Could you check a few things on this model? Use its own coordinates, in mm. Face numbers are marked on the shaded views. A direction names the side the tool comes from. Give positions to 0.01 mm unless a question says otherwise; leave off trailing zeros. Loops run counter-clockwise (first coordinate to the right, second up) from the corner with the lowest first, then second, coordinate; pieces in that order, holes last. Notation, with made-up numbers: (-26.5, 70) - (10.5, 70) arc R27 cw to (10.5, 97) - close; hole circle Ø11 at (32.25, -12.5). An arc over 180 degrees is marked (long way). Write each question's results on one line, items separated by ' | '. Start each with the question number.
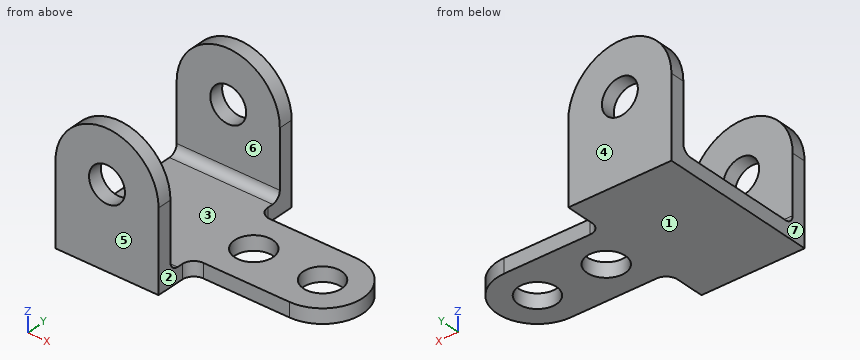
```python
from build123d import *

# Parameters (mm, degrees)
F0_R     = 9.94537
F1_DEPTH = 88.9
F3_DEPTH = 57.151
F4_R     = 10.5537
F5_DEPTH = 7.9375


with BuildPart() as f1:
    # F0 (on Front) → F1 (new body)
    with BuildSketch(Plane.XZ):
        with BuildLine():
            Line((28.575, 0), (28.575, 44.45))
            ThreePointArc((28.575, 44.45), (0, 73.025), (-28.575, 44.45))
            Line((-28.575, 44.45), (-28.575, 0))
            Line((-28.575, 0), (28.575, 0))
        make_face()
        with Locations((0, 44.45)):
            Circle(F0_R, mode=Mode.SUBTRACT)
    extrude(amount=F1_DEPTH)

    # F2 (on face) → F3 (cut, through all)
    with BuildSketch(Plane.YZ.offset(28.575)):
        with BuildLine():
            Line((-7.9375, 77.544321), (-80.9625, 77.544321))
            Line((-80.9625, 77.544321), (-80.9625, 12.7))
            ThreePointArc((-80.9625, 12.7), (-79.567596, 9.332404), (-76.2, 7.9375))
            Line((-76.2, 7.9375), (-12.7127, 7.9375))
            ThreePointArc((-12.7127, 7.9375), (-9.336124, 9.336124), (-7.9375, 12.7127))
            Line((-7.9375, 12.7127), (-7.9375, 77.544321))
        make_face()
    extrude(amount=-F3_DEPTH, mode=Mode.SUBTRACT)

    # F4 (on Top) → F5 (join)
    with BuildSketch(Plane.XY):
        with BuildLine():
            ThreePointArc((34.925, -22.23135), (30.434872, -20.371478), (28.575, -15.88135))
            Line((28.575, -15.88135), (28.575, -73.03135))
            ThreePointArc((28.575, -73.03135), (30.434872, -68.541222), (34.925, -66.68135))
            Line((34.925, -66.68135), (82.55, -66.68135))
            ThreePointArc((82.55, -66.68135), (104.775, -44.45635), (82.55, -22.23135))
            Line((82.55, -22.23135), (34.925, -22.23135))
        make_face()
        with Locations((44.45, -44.45635)):
            Circle(F4_R, mode=Mode.SUBTRACT)
        with Locations((82.55, -44.45635)):
            Circle(F4_R, mode=Mode.SUBTRACT)
    extrude(amount=F5_DEPTH)


solid = f1.part
```
Q1. I want a section at D-D, the plane z = 40. List the corners of the cut face in (x, y) for me (1 decimal).
Q2. I want a section at A-A, the plane x = 0. List the corners of the cut face in (y, z) for me (1 decimal), then the cut area to 3 significant figures.
Q3. I want a section at B-B, the plane x = 44.45. List the corners of the cut face in (y, z) for me.
Q4. I'm going to push flat-ended pins straight in: pin 1 Ø10 at (y, z) = (-28, 16.5) entering from -X; pin 2 Ø8.5 at (x, z) = (68.5, 3.5) entering from -Y; pin 3 Ø12 at (y, z) = (-77, 60.5) entering from +X; pin 4 Ø12.5 at (y, z) = (-84, 29) entering from +X (3 decimals). Where does each tip first touch, or does it pass through?
Q5. I want a section at C-C, the plane z = 22.5. List the corners of the cut face in (x, y) for me (1 decimal).
Q6. If we mould it in two halves opening along Y, with no side actions, what happens to the marked faces 4, 5, 6 and 7? For each: +Y half, -Y half, draft (parallel to the pull), parting line (faces both ways), or undercut.
Q7. Which directions (+Z, -Z, +X, -X, +Y, -Y) give clear straight access to the entire face, cutting with the end or side of a thin tool? Please do the marked faces 1, 2 and 3.
Q8. I need wall thicknesses on L1, parallel to X at y = -84.25, z = 44.45 (3 decimals); L2, parallel to Y at x = -21.5, z = 22; L3, parallel to Y at x = 44, z = 5. Which ranges of each line are inside material? Lowest first, please. Write a range as from..to.
Conclusion:
1) outline: (-28.6, -88.9) - (-8.9, -88.9) - (-8.9, -81) - (-28.6, -81) - close; (-28.6, -7.9) - (-8.9, -7.9) - (-8.9, 0) - (-28.6, 0) - close; (8.9, -88.9) - (28.6, -88.9) - (28.6, -81) - (8.9, -81) - close; (8.9, -7.9) - (28.6, -7.9) - (28.6, 0) - (8.9, 0) - close
2) outline: (-88.9, 0) - (0, 0) - (0, 34.5) - (-7.9, 34.5) - (-7.9, 12.7) arc R4.8 cw to (-12.7, 7.9) - (-76.2, 7.9) arc R4.8 cw to (-81, 12.7) - (-81, 34.5) - (-88.9, 34.5) - close; (-88.9, 54.4) - (-81, 54.4) - (-81, 73) - (-88.9, 73) - close; (-7.9, 54.4) - (0, 54.4) - (0, 73) - (-7.9, 73) - close | area: 1,430 mm^2
3) outline: (-66.68, 0) - (-55.01, 0) - (-55.01, 7.94) - (-66.68, 7.94) - close; (-33.9, 0) - (-22.23, 0) - (-22.23, 7.94) - (-33.9, 7.94) - close
4) pin 1: through | pin 2: y = -66.68 | pin 3: x = 26.14 | pin 4: x = 28.575
5) outline: (-28.6, -88.9) - (28.6, -88.9) - (28.6, -81) - (-28.6, -81) - close; (-28.6, -7.9) - (28.6, -7.9) - (28.6, 0) - (-28.6, 0) - close
6) face 4: +Y half | face 5: -Y half | face 6: undercut | face 7: draft
7) face 1: -Z, +X, -X, +Y, -Y | face 2: +Z, -Z, +X, -Y | face 3: +Z, +X, -X
8) L1: -28.575..-9.945, 9.945..28.575 | L2: -88.9..-80.96, -7.94..0 | L3: -66.68..-55, -33.91..-22.23
